Design review of the part built by this model. Coordinates are the model's own, in mm. A direction names the side the tool comes from. Coordinates: 2 decimals unless noted, no trailing zeros. Order: outer loops, then holes, each group sorted by start corner. A loop starts at its lowest first (then second) coordinate and runs counter-clockwise, first axis right, second up. Notation, with made-up numbers: (-36, -28.75) - (-27, -28.75) arc R16 cw to (-27, -14.75) - close; hole circle Ø11 at (26.25, -32.75). An arc over 180 degrees is marked (long way). Write item = value, one per line. Start each with the question number.
```python
from build123d import *

# Parameters (mm, degrees)
SKETCH2_W               = 127
SKETCH2_H               = 139.7
BOSS_EXTRUDE1_DEPTH     = 12.7
SKETCH4_W               = 12.7
SKETCH4_H               = 3.81
CUT_EXTRUDE1_DEPTH      = 76.2
SKETCH5_W               = 12.7
SKETCH5_H               = 3.81
CUT_EXTRUDE2_DEPTH      = 76.2
MIRROR3_COPY_1_SKETCH_W = 12.7
MIRROR3_COPY_1_SKETCH_H = 3.81
MIRROR3_COPY_1_DEPTH    = 76.2
F_1_4_CLEARANCE_HOLE1_D = 6.7564


with BuildPart() as part:
    # Sketch2 → Boss-Extrude1 (new body)
    with BuildSketch(Plane(origin=(0, 0, 0), x_dir=(1, 0, 0), z_dir=(0, 1, 0))):
        Rectangle(SKETCH2_W, SKETCH2_H)
    extrude(amount=BOSS_EXTRUDE1_DEPTH)

    # Sketch4 → Cut-Extrude1 (cut)
    with BuildSketch(Plane(origin=(63.5, 0, 0), x_dir=(0, 0, -1), z_dir=(1, 0, 0))):
        with Locations((-50.8, 10.795)):
            Rectangle(SKETCH4_W, SKETCH4_H)
    cut_extrude1 = extrude(amount=-CUT_EXTRUDE1_DEPTH, mode=Mode.SUBTRACT)

    # Mirror1: Cut-Extrude1 across plane
    add(cut_extrude1.mirror(Plane.XY), mode=Mode.SUBTRACT)

    # Sketch5 → Cut-Extrude2 (cut)
    with BuildSketch(Plane(origin=(63.5, 0, 0), x_dir=(0, 0, -1), z_dir=(1, 0, 0))):
        with Locations((0, 10.795)):
            Rectangle(SKETCH5_W, SKETCH5_H)
    cut_extrude2 = extrude(amount=-CUT_EXTRUDE2_DEPTH, mode=Mode.SUBTRACT)

    # Mirror3: Cut-Extrude1, Cut-Extrude2 across plane
    add(cut_extrude1.mirror(Plane(origin=(0, 0, 0), x_dir=(0, 0, 1), z_dir=(1, 0, 0))), mode=Mode.SUBTRACT)
    add(cut_extrude2.mirror(Plane(origin=(0, 0, 0), x_dir=(0, 0, 1), z_dir=(1, 0, 0))), mode=Mode.SUBTRACT)

    # Mirror3 copy 1 sketch → Mirror3 copy 1 (cut)
    with BuildSketch(Plane.ZY.offset(63.5)):
        with Locations((-50.8, 10.795)):
            Rectangle(MIRROR3_COPY_1_SKETCH_W, MIRROR3_COPY_1_SKETCH_H)
    extrude(amount=-MIRROR3_COPY_1_DEPTH, mode=Mode.SUBTRACT)

    # 1/4 Clearance Hole1 (through all)
    with Locations(Plane(origin=(0, 0, 0), x_dir=(-1, 0, 0), z_dir=(0, -1, 0))):
        with Locations((-50.8, -50.8), (-50.8, 50.8), (50.8, 50.8), (50.8, -50.8)):
            Hole(F_1_4_CLEARANCE_HOLE1_D / 2)


solid = part.part
```
Item 1: Add section C-C on x = -33. Give the boundary of the cut face in (y, z).
Item 2: For line 1 (Z direction, x = 50.8, y = 5.75); line 2 (X direction, y = 2.75, z = -50.8); line 3 (Z direction, x = 16, y = 9.5), list the stretches that pass through material, from the lowest coordinate up.
Item 3: Add section A-A on z = -50.8. Give the boundary of the cut face in (x, y).
Item 4: Add section B-B on x = -50.8. Give the boundary of the cut face in (y, z).
Item 5: Mouldability with a two-part tool opening along X and no side actions: class faces 1 (the flat face through (63.5, 6, 1)), 2 (the flat face through (-1, 6, -69.85)), 3 (the cylindrical face through (50.07, 4.51, 54.1)) as +X half, -X half, draft (parallel to the pull), parting line (faces both ways), or undercut.
Item 6: For P1, Ø4, axis at x = 7, z = -48.5, coming from the +Y side; P2, Ø5, axis at x = -39.5, z = -41, coming from the -Y side, all flat-tipped, find the tip position at first contact; note any pin that passes through.
Item 7: For faces 4 (the flat face through (-1, 6, 69.85)), 5 (the flat face through (-1, 11, -44.45)), list the 3-axis set-ups (+Z, -Z, +X, -X, +Y, -Y) from which the entire face can be reached by the end or side of a thin tool; tool diameter is ignored.
Worked out:
q1.outline = (0, -69.85) - (12.7, -69.85) - (12.7, -57.15) - (8.89, -57.15) - (8.89, -44.45) - (12.7, -44.45) - (12.7, -6.35) - (8.89, -6.35) - (8.89, 6.35) - (12.7, 6.35) - (12.7, 44.45) - (8.89, 44.45) - (8.89, 57.15) - (12.7, 57.15) - (12.7, 69.85) - (0, 69.85) - close
q2.line_1 = -69.85 to -54.18, -47.42 to 47.42, 54.18 to 69.85
q2.line_2 = -63.5 to -54.18, -47.42 to 47.42, 54.18 to 63.5
q2.line_3 = -69.85 to -57.15, -44.45 to -6.35, 6.35 to 44.45, 57.15 to 69.85
q3.outline = (-63.5, 0) - (-54.18, 0) - (-54.18, 8.89) - (-63.5, 8.89) - close; (-47.42, 0) - (47.42, 0) - (47.42, 8.89) - (-47.42, 8.89) - close; (54.18, 0) - (63.5, 0) - (63.5, 8.89) - (54.18, 8.89) - close
q4.outline = (0, -69.85) - (12.7, -69.85) - (12.7, -57.15) - (8.89, -57.15) - (8.89, -54.18) - (0, -54.18) - close; (0, -47.42) - (8.89, -47.42) - (8.89, -44.45) - (12.7, -44.45) - (12.7, -6.35) - (8.89, -6.35) - (8.89, 6.35) - (12.7, 6.35) - (12.7, 44.45) - (8.89, 44.45) - (8.89, 47.42) - (0, 47.42) - close; (0, 54.18) - (8.89, 54.18) - (8.89, 57.15) - (12.7, 57.15) - (12.7, 69.85) - (0, 69.85) - close
q5.face_1 = +X half
q5.face_2 = draft
q5.face_3 = undercut
q6.P1 = 8.89
q6.P2 = 0
q7.face_4 = +Z, +X, -X, +Y, -Y
q7.face_5 = +X, -X, +Y
